Source: three-view drawing plus pictorial views. Frame: mm from the lowest corner of the part. A direction names the side the tool comes from. Coordinates: 2 decimals unless noted, no trailing zeros. Write each loop counter-clockwise with the first axis right and the second up, starting at its lowest first coordinate (ties: lowest second). Pieces come first, ordered by that corner, then holes. Notation, with made-up numbers: (23.5, -30.5) - (59.5, -30.5) arc R14 ccw to (59.5, -24.5) - close; hole circle Ø2 at (-34.5, -8.5). An arc over 180 degrees is marked (long way). One line per item, written item: value.
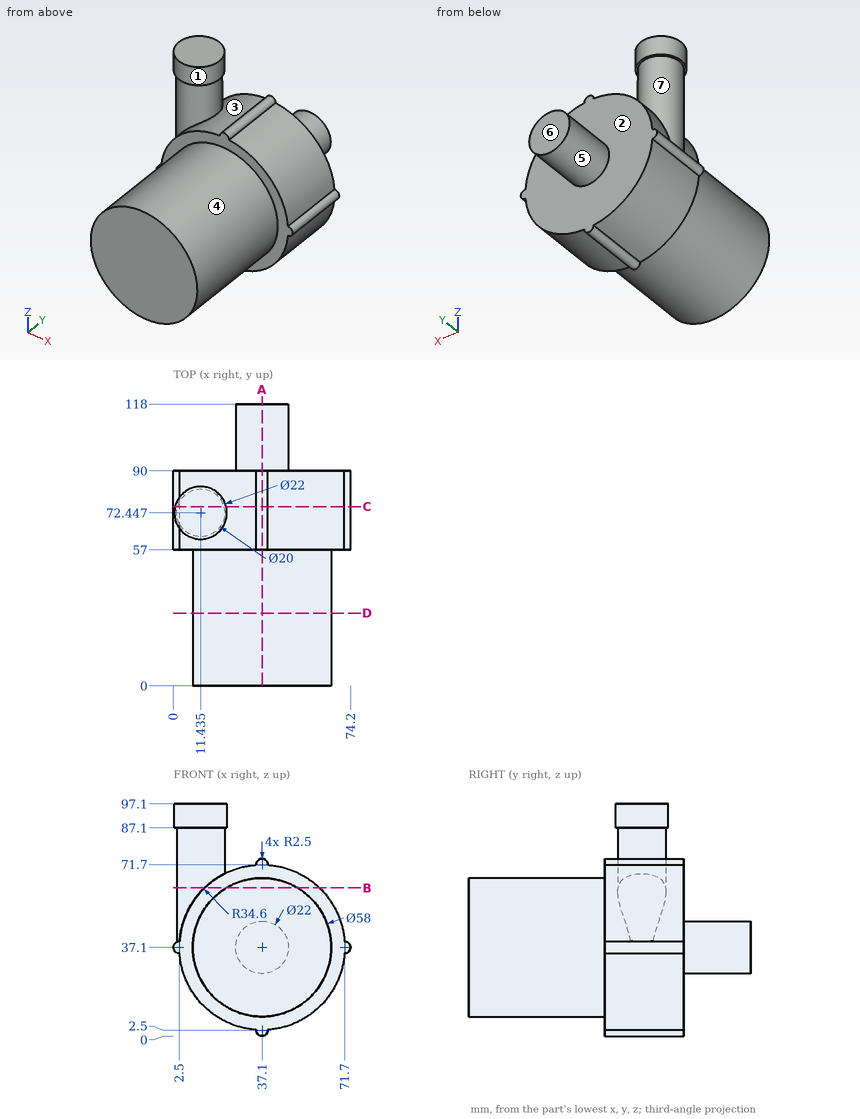
1) Section query C-C on y = 75. Output: boundary loops of the cut face in (x, z) (1 decimal).
Values found:
outline: (0.7, 87.1) - (1.8, 87.1) - (1.8, 39.5) arc R2.5 ccw to (2.6, 34.6) arc R34.6 ccw to (34.6, 2.6) arc R2.5 ccw (long way) to (39.6, 2.6) arc R34.6 ccw to (71.6, 34.6) arc R2.5 ccw (long way) to (71.6, 39.6) arc R34.6 ccw to (39.6, 71.6) arc R2.5 ccw (long way) to (34.6, 71.6) arc R34.6 ccw to (21.1, 67.8) - (21.1, 87.1) - (22.1, 87.1) - (22.1, 97.1) - (0.7, 97.1) - close
2) Draft query along X for the marked faces 5, 6 and 7. Return one class per face: released by +X, released by -X, zero draft, split by the parting line, or undercut.
Values found:
face 5: split by the parting line
face 6: zero draft
face 7: undercut
3) Material intervals for line 1 (Y direction, x = 45, z = 12.5); line 2 (Z direction, x = 21.5, y = 71); line 3 (Y direction, x = 4.5, z = 41.5), sorted ascending.
Values found:
line 1: 0 to 90
line 2: 6.22 to 67.98, 87.1 to 97.1
line 3: 57 to 90
4) Section query D-D on y = 30.5. Output: boundary loops of the cut face in (x, z).
Values found:
outline: circle Ø58 at (37.1, 37.1)
5) Section query B-B on z = 62. Output: boundary loops of the cut face in (x, y) (1 decimal).
Values found:
outline: (13.1, 57) - (22.2, 57) - (22.2, 0) - (52, 0) - (52, 57) - (61.1, 57) - (61.1, 90) - (13.1, 90) - (13.1, 82.3) arc R10 ccw (long way) to (13.1, 62.6) - close
6) Reachability of the marked faces 1, 2, 3 and 4 from +Z, -Z, +X, -X, +Y, -Y: full face, straight path, thin tool, end or side. Return the list, or none.
Values found:
face 1: +Z
face 2: +Y
face 3: none
face 4: -Y
7) Section query A-A on x = 37.1. Output: boundary loops of the cut face in (y, z), then the cut area to 3 significant figures.
Values found:
outline: (0, 8.1) - (57, 8.1) - (57, 0) - (90, 0) - (90, 26.1) - (118, 26.1) - (118, 48.1) - (90, 48.1) - (90, 74.2) - (57, 74.2) - (57, 66.1) - (0, 66.1) - close
area: 6,370 mm2
8) Contact query for flat-ended pins moving along their axis: P1, Ø3, axis at x = 30.5, y = 86.5, coming from the -Z side; P2, Ø8, axis at x = 33, y = 99, coming from the +Z side; P3, Ø6, axis at y = 43, z = 25, coming from the -X side (1 decimal). Output: stop coordinate, or through.
Values found:
P1: z = 2.88
P2: z = 48.1
P3: x = 9.6
